```python
from build123d import *

# Parameters (mm, degrees)
BOSS_EXTRUDE3_DEPTH = 60
SKETCH6_W           = 80
SKETCH6_H           = 5
BOSS_EXTRUDE4_DEPTH = 0.5


with BuildPart() as part:
    # Sketch5 → Boss-Extrude3 (new body)
    with BuildSketch(Plane(origin=(0, 0, 0), x_dir=(1, 0, 0), z_dir=(0, 1, 0))):
        with BuildLine():
            Line((83.381197846, 5), (-83.381197846, 5))
            ThreePointArc((-83.381197846, 5), (-87.381197846, 3.92820323), (-90.309401077, 1))
            Line((-90.309401077, 1), (-90.886751346, 0))
            Line((-90.886751346, 0), (-73.39303819, -10.1))
            Line((-73.39303819, -10.1), (-113.39303819, -79.382032303))
            Line((-113.39303819, -79.382032303), (-109.062911171, -81.882032303))
            Line((-109.062911171, -81.882032303), (-100.124355653, -66.4))
            ThreePointArc((-100.124355653, -66.4), (-96.464101615, -62.739745962), (-91.464101615, -61.4))
            Line((-91.464101615, -61.4), (91.464101615, -61.4))
            ThreePointArc((91.464101615, -61.4), (96.464101615, -62.739745962), (100.124355653, -66.4))
            Line((100.124355653, -66.4), (109.062911171, -81.882032303))
            Line((109.062911171, -81.882032303), (113.39303819, -79.382032303))
            Line((113.39303819, -79.382032303), (73.39303819, -10.1))
            Line((73.39303819, -10.1), (90.886751346, 0))
            Line((90.886751346, 0), (90.309401077, 1))
            ThreePointArc((90.309401077, 1), (87.381197846, 3.92820323), (83.381197846, 5))
        make_face()
        with BuildLine():
            Line((7.1, -20.4), (-7.1, -20.4))
            ThreePointArc((-7.1, -20.4), (-7.453553391, -20.253553391), (-7.6, -19.9))
            Line((-7.6, -19.9), (-7.6, -18.9))
            ThreePointArc((-7.6, -18.9), (-7.746446609, -18.546446609), (-8.1, -18.4))
            Line((-8.1, -18.4), (-12.1, -18.4))
            ThreePointArc((-12.1, -18.4), (-12.453553391, -18.546446609), (-12.6, -18.9))
            Line((-12.6, -18.9), (-12.6, -19.9))
            ThreePointArc((-12.6, -19.9), (-12.746446609, -20.253553391), (-13.1, -20.4))
            Line((-13.1, -20.4), (-18.7, -20.4))
            ThreePointArc((-18.7, -20.4), (-19.760660172, -19.960660172), (-20.2, -18.9))
            Line((-20.2, -18.9), (-20.2, -1.5))
            ThreePointArc((-20.2, -1.5), (-19.760660172, -0.439339828), (-18.7, 0))
            Line((-18.7, 0), (-13.1, 0))
            ThreePointArc((-13.1, 0), (-12.746446609, -0.146446609), (-12.6, -0.5))
            Line((-12.6, -0.5), (-12.6, -1.5))
            ThreePointArc((-12.6, -1.5), (-12.453553391, -1.853553391), (-12.1, -2))
            Line((-12.1, -2), (-8.1, -2))
            ThreePointArc((-8.1, -2), (-7.746446609, -1.853553391), (-7.6, -1.5))
            Line((-7.6, -1.5), (-7.6, -0.5))
            ThreePointArc((-7.6, -0.5), (-7.453553391, -0.146446609), (-7.1, 0))
            Line((-7.1, 0), (7.1, 0))
            ThreePointArc((7.1, 0), (7.453553391, -0.146446609), (7.6, -0.5))
            Line((7.6, -0.5), (7.6, -1.5))
            ThreePointArc((7.6, -1.5), (7.746446609, -1.853553391), (8.1, -2))
            Line((8.1, -2), (12.1, -2))
            ThreePointArc((12.1, -2), (12.453553391, -1.853553391), (12.6, -1.5))
            Line((12.6, -1.5), (12.6, -0.5))
            ThreePointArc((12.6, -0.5), (12.746446609, -0.146446609), (13.1, 0))
            Line((13.1, 0), (18.7, 0))
            ThreePointArc((18.7, 0), (19.760660172, -0.439339828), (20.2, -1.5))
            Line((20.2, -1.5), (20.2, -18.9))
            ThreePointArc((20.2, -18.9), (19.760660172, -19.960660172), (18.7, -20.4))
            Line((18.7, -20.4), (13.1, -20.4))
            ThreePointArc((13.1, -20.4), (12.746446609, -20.253553391), (12.6, -19.9))
            Line((12.6, -19.9), (12.6, -18.9))
            ThreePointArc((12.6, -18.9), (12.453553391, -18.546446609), (12.1, -18.4))
            Line((12.1, -18.4), (8.1, -18.4))
            ThreePointArc((8.1, -18.4), (7.746446609, -18.546446609), (7.6, -18.9))
            Line((7.6, -18.9), (7.6, -19.9))
            ThreePointArc((7.6, -19.9), (7.453553391, -20.253553391), (7.1, -20.4))
        make_face(mode=Mode.SUBTRACT)
        with BuildLine():
            Line((-71.256842194, -26.4), (71.256842194, -26.4))
            ThreePointArc((71.256842194, -26.4), (76.256842194, -27.739745962), (79.917096231, -31.4))
            Line((79.917096231, -31.4), (90.598076211, -49.9))
            ThreePointArc((90.598076211, -49.9), (90.598076211, -54.9), (86.267949192, -57.4))
            Line((86.267949192, -57.4), (-86.267949192, -57.4))
            ThreePointArc((-86.267949192, -57.4), (-90.598076211, -54.9), (-90.598076211, -49.9))
            Line((-90.598076211, -49.9), (-79.917096231, -31.4))
            ThreePointArc((-79.917096231, -31.4), (-76.256842194, -27.739745962), (-71.256842194, -26.4))
        make_face(mode=Mode.SUBTRACT)
    extrude(amount=BOSS_EXTRUDE3_DEPTH)

    # Sketch6 → Boss-Extrude4 (add)
    with BuildSketch(Plane(origin=(-50.671350353, 0, -29.255117767), x_dir=(-0.5, 0, 0.866025404), z_dir=(-0.866025404, 0, -0.5))):
        with Locations((85.443375673, 50)):
            Rectangle(SKETCH6_W, SKETCH6_H)
        with Locations((85.443375673, 10)):
            Rectangle(SKETCH6_W, SKETCH6_H)
    extrude(amount=BOSS_EXTRUDE4_DEPTH)


solid = part.part
```
Can you work these out from the model? Positions are in its coordinate system, mm. A direction names the side the tool comes from. Coordinates: 2 decimals unless noted, no trailing zeros. Loops run counter-clockwise (first coordinate to the right, second up) from the corner with the lowest first, then second, coordinate; pieces in that order, holes last.
1) Imagine slicing it at D-D on z = 4.5. List the corners of the cut face in (x, y) for me.
2) Imagine slicing it at B-B on z = 53. List the corners of the cut face in (x, y) for me.
3) Imagine slicing it at C-C on y = 4.5. State how many separate pieces and enclosed holes the cut face has, plus the area to 3 significant figures.
4) Imagine slicing it at A-A on x = -63. List the corners of the cut face in (y, z) for me.
5) Thinking about a two-plate mould opening in Y: for faces 4 (the flat face through (-93.3, 52.5, 44.1)), 5 (the flat face through (-93.3, 12.5, 44.1)), 6 (the flat face through (-104.656, 29.58, 74.249)), which applies, pulls with the +Y half, pulls with the -Y half, needs draft (parallel to the pull), parting line crosses it, or undercut?
6) I need wall thicknesses on probe 1 along Z at (x, y) = (-12, 47); probe 2 along Z at (x, y) = (28, 13); probe 3 along Z at (x, y) = (-17, 36.5). Which ranges of each line are inside material? Lowest first, please.
7) Which directions (+Z, -Z, +X, -X, +Y, -Y) give clear straight access to the entire face, cutting with the end or side of a thin tool? Please do faces 1 (the flat face through (104.53, 29.58, 74.03)), 2 (the flat face through (16, 30, 0)), 3 (the flat face through (82.02, 29.58, 5.12)).
8) For pin 1 (1.1 mm diameter, centred on y = 29.5, z = 19.5, fed in from +X); pin 2 (2 mm diameter, centred on x = 78, z = 63, fed in from -Y); pin 3 (1.7 mm diameter, centred on x = 17, y = 19, fed in from +Z); pin 4 (2 mm diameter, centred on y = 9, z = 55.5, fed in from -X), each with a flat end and sliding along its axis, tell me the tip position at first contact or that it passes through.
Completed:
1. outline: (-83.09, 0) - (-20.2, 0) - (-20.2, 60) - (-83.09, 60) - close; (20.2, 0) - (83.09, 0) - (83.09, 60) - (20.2, 60) - close
2. outline: (-98.74, 7.5) - (-98.16, 7.5) - (-98.16, 0) - (-91.23, 0) - (-91.23, 60) - (-98.16, 60) - (-98.16, 52.5) - (-98.74, 52.5) - (-98.74, 47.5) - (-98.16, 47.5) - (-98.16, 12.5) - (-98.74, 12.5) - close; (91.23, 0) - (98.16, 0) - (98.16, 60) - (91.23, 60) - close
3. separate pieces: 1
3. enclosed holes: 2
3. area: 5,760 mm2
4. outline: (0, -5) - (60, -5) - (60, 26.4) - (0, 26.4) - close; (0, 57.4) - (60, 57.4) - (60, 61.4) - (0, 61.4) - close
5. face 4: pulls with the +Y half
5. face 5: undercut
5. face 6: needs draft
6. probe 1: z = -5 to 2, 18.4 to 26.4, 57.4 to 61.4
6. probe 2: z = -5 to 26.4, 57.4 to 61.4
6. probe 3: z = -5 to 0, 20.4 to 26.4, 57.4 to 61.4
7. face 1: +Z, +Y, -Y
7. face 2: +Y, -Y
7. face 3: +X, +Y, -Y
8. pin 1: stops at x = 79.14
8. pin 2: passes through
8. pin 3: stops at z = 61.4
8. pin 4: stops at x = -100.76
